```python
from build123d import *

# Parameters (mm, degrees)
SKETCH002_R      = 1.5
EXTRUDE002_DEPTH = 10
SKETCH_W         = 200
SKETCH_H         = 20
EXTRUDE_DEPTH    = 3
FACE001_W        = 5
FACE001_H        = 200
EXTRUDE001_DEPTH = 10


with BuildPart() as extrude002:
    # Sketch002 (on Face6 of Extrude) → Extrude002 (new body)
    with BuildSketch(Plane.XY.offset(3)):
        with Locations((50, 12.5)):
            Circle(SKETCH002_R)
        with Locations((150, 12.5)):
            Circle(SKETCH002_R)
    extrude(amount=-EXTRUDE002_DEPTH)


with BuildPart() as cut:
    # Sketch → Extrude (new body)
    with BuildSketch(Plane.XY):
        with Locations((100, 10)):
            Rectangle(SKETCH_W, SKETCH_H)
    extrude(amount=EXTRUDE_DEPTH)

    # Cut: cut Extrude002
    add(extrude002.part, mode=Mode.SUBTRACT)


with BuildPart() as fusion:
    # Face001 → Extrude001 (new body)
    with BuildSketch(Plane(origin=(100, 2.5, 3), x_dir=(0, 1, 0), z_dir=(0, 0, 1))):
        Rectangle(FACE001_W, FACE001_H)
    extrude(amount=EXTRUDE001_DEPTH)

    # Fusion: union Cut
    add(cut.part)


solid = fusion.part
```
Model file for the job. Use its own axes, mm. A direction names the side the tool comes from. Give positions to 0.01 mm unless a question says otherwise; leave off trailing zeros. Order: outer loops, then holes, each group sorted by start corner. A loop starts at its lowest first (then second) coordinate and runs counter-clockwise, first axis right, second up.
1) 3-axis set-ups, long thin cutter, end or side, ignore diameter. For faces 1 (the flat face through (101, 5, 8)), 2 (the flat face through (200, 5, 2)): which of +Z, -Z, +X, -X, +Y, -Y reach the whole face in a straight line?
2) Saw through at C-C, the plane y = 17.25. Write the cut outline in (x, z), then the cut area to 3 significant figures.
3) Saw through at A-A, the plane x = 138. Write the cut outline in (y, z), then the cut area to 3 significant figures.
4) Saw through at B-B, the plane z = 6. Write the cut outline in (x, y).
5) Pin check, flat tips, straight feed: pin 1 (1 mm diameter, centred on x = 68, y = 5, fed in from -Z); pin 2 (12 mm diameter, centred on x = 137.5, y = 14, fed in from +Z); pin 3 (3 mm diameter, centred on x = 159, z = 7.5, fed in from +Y). Stop position of each tip, or through.
6) Wall check: probe 1 along Y at (x, z) = (50, 0.95); probe 2 along Z at (x, y) = (17.5, 7); probe 3 along Y at (x, z) = (97, 3.25). Give the ranges that are in metal, low to high.
Computed:
1. face 1: +Z, +X, -X, +Y
1. face 2: +Z, -Z, +X, +Y, -Y
2. outline: (0, 0) - (200, 0) - (200, 3) - (0, 3) - close
2. area: 600 mm2
3. outline: (0, 0) - (20, 0) - (20, 3) - (5, 3) - (5, 13) - (0, 13) - close
3. area: 110 mm2
4. outline: (0, 0) - (200, 0) - (200, 5) - (0, 5) - close
5. pin 1: stops at z = 0
5. pin 2: stops at z = 3
5. pin 3: stops at y = 5
6. probe 1: y = 0 to 11, 14 to 20
6. probe 2: z = 0 to 3
6. probe 3: y = 0 to 5
